from build123d import *

# Parameters (mm, degrees)
SKETCH14_R         = 4
CUT_EXTRUDE2_DEPTH = 10


with BuildPart() as part:
    # Sketch1 → Revolve2 (revolve)
    with BuildSketch(Plane.XY):
        Polygon((14, 0.233571738), (38.150093927, 0.233571738), (38.150093927, 10.233571738), (21, 10.233571738), (21, 15.233571738), (16.5, 15.233571738), (16.5, 10.233571738), (14, 10.233571738), align=None)
    revolve(axis=Axis((0, 0, 0), (0, 1, 0)))

    # Sketch14 → Cut-Extrude2 (cut)
    with BuildSketch(Plane(origin=(0, 10.233571738, 0), x_dir=(1, 0, 0), z_dir=(0, 1, 0))):
        with Locations((25, 0)):
            Circle(SKETCH14_R)
        with Locations((0, 25)):
            Circle(SKETCH14_R)
        with Locations((-25, 0)):
            Circle(SKETCH14_R)
        with Locations((0, -25)):
            Circle(SKETCH14_R)
    extrude(amount=-CUT_EXTRUDE2_DEPTH, mode=Mode.SUBTRACT)


solid = part.part
Part model, mm, in its own coordinate system. A direction names the side the tool comes from. Give positions to 0.01 mm unless a question says otherwise; leave off trailing zeros. Order: outer loops, then holes, each group sorted by start corner. A loop starts at its lowest first (then second) coordinate and runs counter-clockwise, first axis right, second up. Notation, with made-up numbers: (30.25, -30.75) - (45.25, -30.75) arc R11 ccw to (45.25, -22.75) - close; hole circle Ø3 at (14.25, 50). An arc over 180 degrees is marked (long way). Use a Markdown table: item, result.
1) 3-axis set-ups, long thin cutter, end or side, ignore diameter. For faces 1 (the cylindrical face through (21.8, 5.3, 2.4)), 2 (the flat face through (16, 10.234, 16)): which of +Z, -Z, +X, -X, +Y, -Y reach the whole face in a straight line?
Checked values:
| item | result |
|---|---|
| face 1 | +Y, -Y |
| face 2 | +Y |
2) Saw through at D-D on z = -18.5. List the corners of the cut face in (x, y).
Checked values:
| item | result |
|---|---|
| outline | (-33.36, 0.23) - (33.36, 0.23) - (33.36, 10.23) - (9.94, 10.23) - (9.94, 15.23) - (-9.94, 15.23) - (-9.94, 10.23) - (-33.36, 10.23) - close |
3) Flat gauge pins, fed straight in: P1, Ø2, axis at x = -23.5, y = 4.5, coming from the +Z side; P2, Ø9, axis at x = 0, z = -25, coming from the +Y side; P3, Ø6, axis at y = 3, z = 19, coming from the -X side; P4, Ø3, axis at x = 15.5, y = 11.5, coming from the -Z side. Where does each tip first touch, or does it go through?
Checked values:
| item | result |
|---|---|
| P1 | z = 30.81 |
| P2 | y = 15.23 |
| P3 | x = -34.63 |
| P4 | z = -35.21 |
4) Saw through at C-C on x = -13. List the corners of the cut face in (y, z).
Checked values:
| item | result |
|---|---|
| outline | (0.23, -35.87) - (10.23, -35.87) - (10.23, -16.49) - (15.23, -16.49) - (15.23, -10.16) - (10.23, -10.16) - (10.23, -5.2) - (0.23, -5.2) - close; (0.23, 5.2) - (10.23, 5.2) - (10.23, 10.16) - (15.23, 10.16) - (15.23, 16.49) - (10.23, 16.49) - (10.23, 35.87) - (0.23, 35.87) - close |
5) Saw through at A-A on y = 4.75. List the corners of the cut face in (x, z), plus the area to 3 significant figures.
Checked values:
| item | result |
|---|---|
| outline | circle Ø76.3 at (0, 0); hole circle Ø8 at (-25, 0); hole circle Ø28 at (0, 0); hole circle Ø8 at (0, -25); hole circle Ø8 at (0, 25); hole circle Ø8 at (25, 0) |
| area | 3,760 mm² |
6) Probe L1, parallel to Z at x = 0, y = 4.75; L2, parallel to X at y = 13.9, z = 0. List the from-to ranges inside material, lowest first. Write a range as from..to.
Checked values:
| item | result |
|---|---|
| L1 | -38.15..-29, -21..-14, 14..21, 29..38.15 |
| L2 | -21..-16.5, 16.5..21 |
7) Saw through at B-B on z = 25. List the corners of the cut face in (x, y).
Checked values:
| item | result |
|---|---|
| outline | (-28.82, 0.23) - (-4, 0.23) - (-4, 10.23) - (-28.82, 10.23) - close; (4, 0.23) - (28.82, 0.23) - (28.82, 10.23) - (4, 10.23) - close |
